from build123d import *

# Parameters (mm, degrees)
SKETCH1_W           = 4.1
SKETCH1_H           = 1.7
BOSS_EXTRUDE1_DEPTH = 1.5


with BuildPart() as part:
    # Sketch1 → Boss-Extrude1 (new body)
    with BuildSketch(Plane(origin=(0, 0, 0), x_dir=(1, 0, 0), z_dir=(0, 1, 0))):
        Polygon((3.75, 30), (5.75, 30), (5.75, -14.9), (4.25, -14.9), (4.25, -16.6), (5.75, -16.6), (5.75, -30), (3.75, -30), (3.75, -31.5), (-3.75, -31.5), (-3.75, -30), (-5.75, -30), (-5.75, -16.6), (-4.25, -16.6), (-4.25, -14.9), (-5.75, -14.9), (-5.75, 30), (-3.75, 30), (-3.75, 31.5), (3.75, 31.5), align=None)
        with Locations((0, 18.65)):
            Rectangle(SKETCH1_W, SKETCH1_H, mode=Mode.SUBTRACT)
    extrude(amount=BOSS_EXTRUDE1_DEPTH)


solid = part.part
Design review of the part built by this model. Coordinates are the model's own, in mm. A direction names the side the tool comes from. Coordinates: 2 decimals unless noted, no trailing zeros. Loops run counter-clockwise (first coordinate to the right, second up) from the corner with the lowest first, then second, coordinate; pieces in that order, holes last. Notation, with made-up numbers: (-4.75, 9.5) - (54.25, 9.5) arc R14 ccw to (54.25, 22.5) - close; hole circle Ø11 at (-25, 25.5). An arc over 180 degrees is marked (long way). Use CSV: the item, a comma, the result in double quotes. Start each with the question number.
1. Mouldability with a two-part tool opening along X and no side actions: class faces 1 (the flat face through (3.75, 1, -31)), 2 (the flat face through (2.05, 1, -19)), 3 (the flat face through (0, 1, 31.5)) as released by +X, released by -X, zero draft, split by the parting line, or undercut.
2. Clearance check with flat-ended pins moving along their axes: pin 1 (0.8 mm diameter, centred on x = 5, y = 1, fed in from -Z); pin 2 (0.8 mm diameter, centred on y = 0.5, z = -30.5, fed in from -X); pin 3 (0.8 mm diameter, centred on x = -5, y = 1, fed in from +Z). State where each tip first meets the part, or that it passes through.
3. Add section A-A on x = -1.25. Give the boundary of the cut face in (y, z), plus the area to 4 significant figures.
4. For faces 4 (the flat face through (5, 1, -30)), 5 (the flat face through (3.75, 1, 31)), 6 (the flat face through (-5, 1, 30)), 7 (the flat face through (4.25, 1, 16)), 8 (the flat face through (-4.25, 1, 16)), list the 3-axis set-ups (+Z, -Z, +X, -X, +Y, -Y) from which the entire face can be reached by the end or side of a thin tool; tool diameter is ignored.
5. Add section B-B on y = 1.2. Give the boundary of the cut face in (x, z).
6. To check wall thickness, follow probe 1 along Z at (x, y) = (4.75, 0.3); probe 2 along Z at (x, y) = (0, 0.1); probe 3 along Z at (x, y) = (-4, 1.05). State the ranges of each line that lie inside material, in increasing order.
Resolved:
1,face 1,"released by +X"
1,face 2,"undercut"
1,face 3,"zero draft"
2,pin 1,"z = -30"
2,pin 2,"x = -3.75"
2,pin 3,"z = 30"
3,outline,"(0, -31.5) - (1.5, -31.5) - (1.5, -19.5) - (0, -19.5) - close; (0, -17.8) - (1.5, -17.8) - (1.5, 31.5) - (0, 31.5) - close"
3,area,"91.95 mm2"
4,face 4,"-Z, +X, +Y, -Y"
4,face 5,"+Z, +X, +Y, -Y"
4,face 6,"+Z, -X, +Y, -Y"
4,face 7,"+X, +Y, -Y"
4,face 8,"-X, +Y, -Y"
5,outline,"(-5.75, -30) - (-3.75, -30) - (-3.75, -31.5) - (3.75, -31.5) - (3.75, -30) - (5.75, -30) - (5.75, 14.9) - (4.25, 14.9) - (4.25, 16.6) - (5.75, 16.6) - (5.75, 30) - (3.75, 30) - (3.75, 31.5) - (-3.75, 31.5) - (-3.75, 30) - (-5.75, 30) - (-5.75, 16.6) - (-4.25, 16.6) - (-4.25, 14.9) - (-5.75, 14.9) - close; hole (-2.05, -19.5) - (2.05, -19.5) - (2.05, -17.8) - (-2.05, -17.8) - close"
6,probe 1,"-30 to 14.9, 16.6 to 30"
6,probe 2,"-31.5 to -19.5, -17.8 to 31.5"
6,probe 3,"-30 to 30"
